Geometry check sheet. Reference: drawing and pictorial views, mm from the part's lowest x, y, z. Give positions to 0.01 mm unless a question says otherwise; leave off trailing zeros. Order: outer loops, then holes, each group sorted by start corner. A loop starts at its lowest first (then second) coordinate and runs counter-clockwise, first axis right, second up. Notation, with made-up numbers: (-24, -32) - (-11, -32) arc R23 cw to (-11, -23) - close; hole circle Ø10 at (71, 73). An arc over 180 degrees is marked (long way). Answer as a JSON object with one key per item and string values.
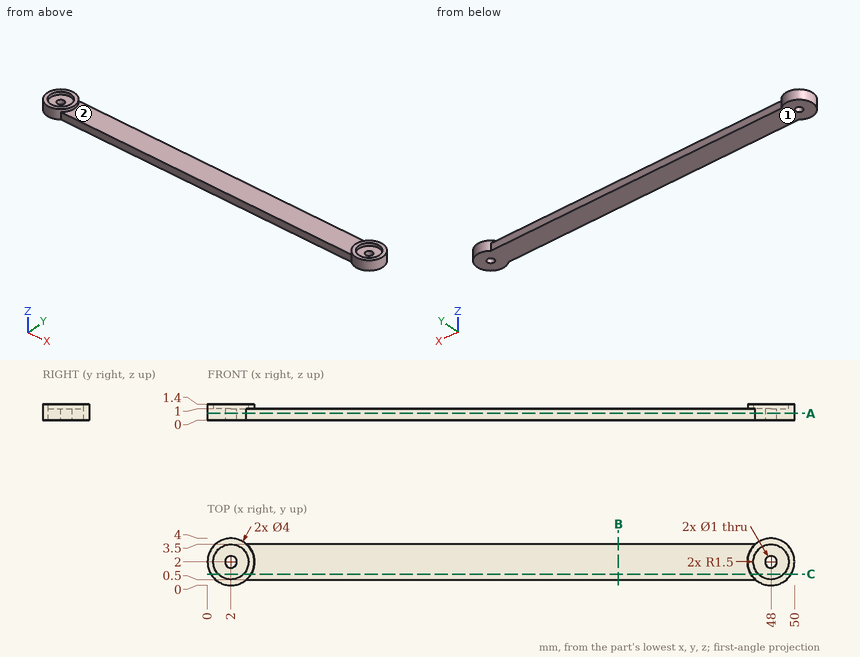
(1) Release check for a two-part mould opening along X. For the marked faces 1 and 2 record: pulls with the +X half, pulls with the -X half, needs draft (parallel to the pull), parting line crosses it, or undercut.
Computed values:
{"face 1": "needs draft", "face 2": "undercut"}
(2) Section check B-B (x = 35). Record the cut outline in (y, z).
Computed values:
{"outline": "(0.5, 0) - (3.5, 0) - (3.5, 1) - (0.5, 1) - close"}
(3) Gauge pin test, flat ends, axial feed: pin 1 Ø0.8 at (x, z) = (26.5, 0.5) entering from -Y; pin 2 Ø1.5 at (x, y) = (1.5, 1.5) entering from +Z. Record the tip position at first contact, or that the pin passes through.
Computed values:
{"pin 1": "stops at y = 0.5", "pin 2": "stops at z = 1"}
(4) Section check C-C (y = 0.95). Record the cut outline in (x, z).
Computed values:
{"outline": "(0.3, 0) - (49.7, 0) - (49.7, 1.4) - (49.07, 1.4) - (49.07, 1) - (46.93, 1) - (46.93, 1.4) - (46.3, 1.4) - (46.3, 1) - (3.7, 1) - (3.7, 1.4) - (3.07, 1.4) - (3.07, 1) - (0.93, 1) - (0.93, 1.4) - (0.3, 1.4) - close"}
(5) Material ranges on line 1 along Y through (x, z) = (2, 0.6); line 2 along X through (y, z) = (1.2, 1.25); line 3 along X through (y, z) = (2.4, 0.15), recorded low to high. Write a range as [from, to].
Computed values:
{"line 1": "y = [0, 1.5], [2.5, 4]", "line 2": "x = [0.17, 0.73], [3.27, 3.83], [46.17, 46.73], [49.27, 49.83]", "line 3": "x = [0.04, 1.7], [2.3, 47.7], [48.3, 49.96]"}
(6) Section check A-A (z = 0.6). Record the cut outline in (x, y), then the cut area to 3 significant figures.
Computed values:
{"outline": "(3.32, 0.5) - (46.68, 0.5) arc R2 ccw (long way) to (46.68, 3.5) - (3.32, 3.5) arc R2 ccw (long way) to start; hole circle Ø1 at (2, 2); hole circle Ø1 at (48, 2)", "area": "151 mm²"}
